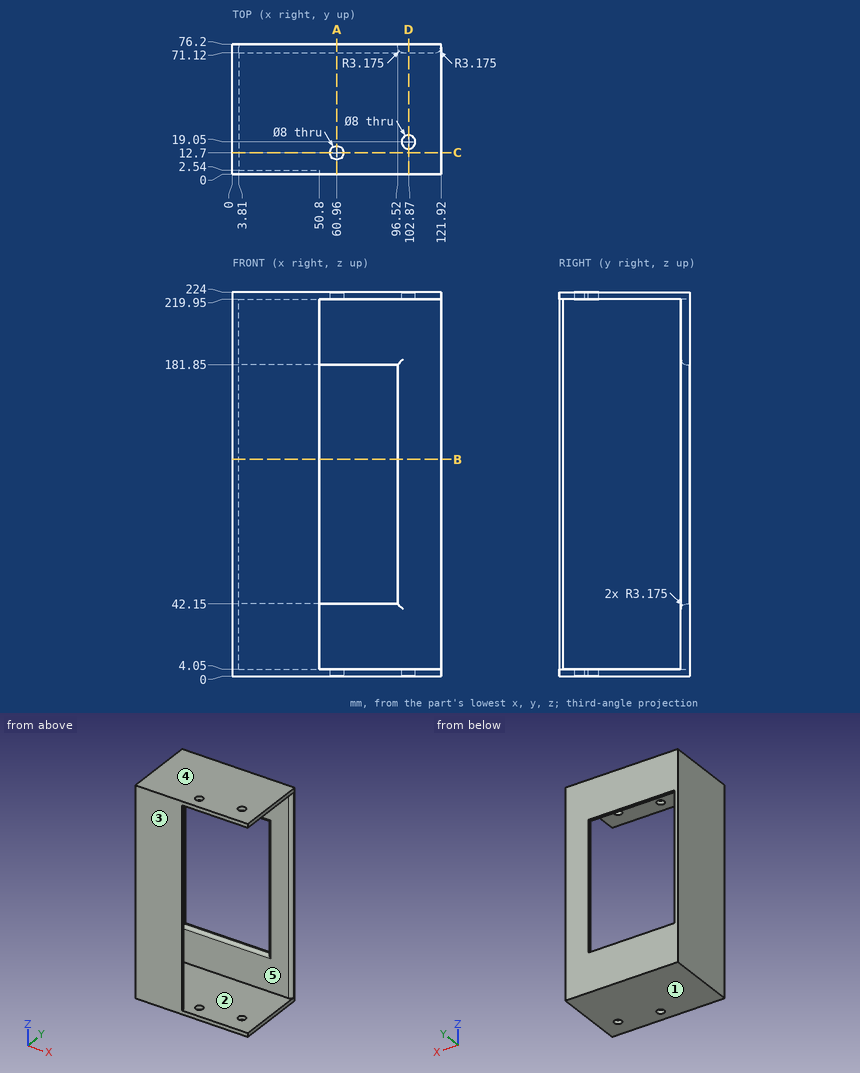
The drawing under review shows one solid part. Ordinate dimensions are in mm from its lowest x, y, z. A direction names the side the tool comes from. Round coordinates to 2 decimals unless told otherwise and drop trailing zeros. Write each loop counter-clockwise with the first axis right and the second up, starting at its lowest first coordinate (ties: lowest second). Pieces come first, ordered by that corner, then holes. Notation, with made-up numbers: (23.5, -9) - (27.5, -9) arc R17 cw to (27.5, 18) - close; hole circle Ø4 at (-18.75, 85). An arc over 180 degrees is marked (long way). Use a Markdown table: item, result. Add a question column.
1. Clearance check with flat-ended pins moving along their axes: pin 1 (14 mm diameter, centred on x = 18.5, z = 93.5, fed in from +Y); pin 2 (1.3 mm diameter, centred on y = 1.5, z = 107, fed in from +X). State where each tip first meets the part, or that it passes through.
2. We need section C-C (y = 12.7). State the section outline as (x, z) points.
3. Wall thickness on probe 1 along Z at (x, y) = (81, 56); probe 2 along X at (y, z) = (19.05, 1.3); probe 3 along X at (y, z) = (12.7, 221): over which ranges is each line inside the solid? List them lowest first.
4. For the marked faces 4 and 5, list the 3-axis set-ups (+Z, -Z, +X, -X, +Y, -Y) from which the entire face can be reached by the end or side of a thin tool; tool diameter is ignored.
5. We need section B-B (z = 126.5). State the section outline as (x, y) points (3 decimals), then the cut area to 3 significant figures.
6. We need section A-A (x = 60.96). State the section outline as (y, z) points (3 decimals), then the cut area to 3 significant figures.
7. Mouldability with a two-part tool opening along Z and no side actions: class the marked faces 1, 2 and 3 as +Z half, -Z half, draft (parallel to the pull), parting line (faces both ways), or undercut.
8. We need section D-D (x = 102.87). State the section outline as (y, z) points.
Output:
| question | item | result |
|---|---|---|
| 1 | pin 1 | stops at y = 2.54 |
| 1 | pin 2 | stops at x = 50.8 |
| 2 | outline | (0, 0) - (56.96, 0) - (56.96, 4.05) - (3.81, 4.05) - (3.81, 219.95) - (56.96, 219.95) - (56.96, 224) - (0, 224) - close; (64.96, 0) - (121.92, 0) - (121.92, 4.05) - (64.96, 4.05) - close; (64.96, 219.95) - (121.92, 219.95) - (121.92, 224) - (64.96, 224) - close |
| 3 | probe 1 | z = 0 to 4.05, 219.95 to 224 |
| 3 | probe 2 | x = 0 to 98.87, 106.87 to 121.92 |
| 3 | probe 3 | x = 0 to 56.96, 64.96 to 121.92 |
| 4 | face 4 | +Z, +X, -X, +Y, -Y |
| 4 | face 5 | +X |
| 5 | outline | (0, 0) - (50.8, 0) - (50.8, 2.54) - (3.81, 2.54) - (3.81, 76.2) - (0, 76.2) - close; (96.52, 74.295) arc R3.175 ccw to (99.695, 71.12) - (118.745, 71.12) arc R3.175 ccw to (121.92, 74.295) - (121.92, 76.2) - (96.52, 76.2) - close |
| 5 | area | 534 mm2 |
| 6 | outline | (0, 0) - (8.7, 0) - (8.7, 4.05) - (0, 4.05) - close; (0, 219.95) - (8.7, 219.95) - (8.7, 224) - (0, 224) - close; (16.7, 0) - (76.2, 0) - (76.2, 42.15) - (74.295, 42.15) arc R3.175 ccw to (71.12, 38.975) - (71.12, 4.05) - (16.7, 4.05) - close; (16.7, 219.95) - (71.12, 219.95) - (71.12, 185.025) arc R3.175 ccw to (74.295, 181.85) - (76.2, 181.85) - (76.2, 224) - (16.7, 224) - close |
| 6 | area | 935 mm2 |
| 7 | face 1 | -Z half |
| 7 | face 2 | undercut |
| 7 | face 3 | draft |
| 8 | outline | (0, 0) - (15.05, 0) - (15.05, 4.05) - (0, 4.05) - close; (0, 219.95) - (15.05, 219.95) - (15.05, 224) - (0, 224) - close; (23.05, 0) - (76.2, 0) - (76.2, 224) - (23.05, 224) - (23.05, 219.95) - (71.12, 219.95) - (71.12, 4.05) - (23.05, 4.05) - close |
